Geometry check sheet. Reference: the model listing, model coordinates, mm. Coordinates: 2 decimals unless noted, no trailing zeros. Order: outer loops, then holes, each group sorted by start corner. A loop starts at its lowest first (then second) coordinate and runs counter-clockwise, first axis right, second up. Notation, with made-up numbers: (-20.75, 74.5) - (11.25, 74.5) arc R23 ccw to (11.25, 101.5) - close; hole circle Ø2 at (-38, 58). An arc over 180 degrees is marked (long way). Return JSON: item names as keys, results as strings. Group by question number.
Item 1: Section check C-C on y = 194.5. Enter the section's corners in (x, z), then the cut area to 3 significant figures.
Item 2: Scan lines: probe 1 along X at (y, z) = (213, 2.9); probe 2 along X at (y, z) = (212, 2.55); probe 3 along X at (y, z) = (192, 0.5). Record each from-to range of solid material in increasing order.
Item 3: Gauge pin test, flat end, axial feed: pin 1 (1.5 mm diameter, centred on y = 207.5, z = 3, fed in from -X). Record the tip position at first contact, or that the pin passes through.
Item 4: Section check B-B on x = 455.25. Enter the section's corners in (y, z), then the cut area to 3 significant figures.
from build123d import *

# Parameters (mm, degrees)
BOSS_EXTRUDE1_DEPTH = 6


with BuildPart() as part:
    # Sketch1 → Boss-Extrude1 (new body)
    with BuildSketch(Plane.XY):
        Polygon((457.663031463, 187.980636569), (464.304980239, 187.980636569), (469.367845751, 193.043502081), (467.079834781, 212.013718005), (466.481000515, 216.863814529), (465.31762376, 218.027191284), (456.81762376, 218.027191284), (455.685560331, 216.895127855), (452.59487335, 193.048794682), align=None)
        Polygon((461.066361502, 210.209676022), (460.599441079, 210.271147261), (460.16434051, 210.451371818), (459.790711182, 210.738067685), (459.504015315, 211.111697013), (459.323790759, 211.546797582), (459.262319519, 212.013718005), (459.323790759, 212.480638429), (459.504015315, 212.915738997), (459.790711182, 213.289368326), (460.16434051, 213.576064193), (460.599441079, 213.756288749), (461.066361502, 213.817759989), (461.533281926, 213.756288749), (461.968382494, 213.576064193), (462.342011823, 213.289368326), (462.62870769, 212.915738997), (462.808932246, 212.480638429), (462.870403486, 212.013718005), (462.808932246, 211.546797582), (462.62870769, 211.111697013), (462.342011823, 210.738067685), (461.968382494, 210.451371818), (461.533281926, 210.271147261), align=None, mode=Mode.SUBTRACT)
    extrude(amount=BOSS_EXTRUDE1_DEPTH)


solid = part.part
Computed:
{
 "1": {"outline": "(452.78, 0) - (469.19, 0) - (469.19, 6) - (452.78, 6) - close", "area": "98.5 mm²"},
 "2": {"probe 1": "x = 455.18 to 459.57, 462.56 to 466.96", "probe 2": "x = 455.05 to 459.26, 462.87 to 467.08", "probe 3": "x = 453.64 to 468.32"},
 "3": {"pin 1": "stops at x = 454.37"},
 "4": {"outline": "(190.39, 0) - (213.53, 0) - (213.53, 6) - (190.39, 6) - close", "area": "139 mm²"}
}
